from build123d import *

# Parameters (mm, degrees)
CROQUIS2_R                                           = 170
CROQUIS2_R_2                                         = 150
CROQUIS2_R_3                                         = 67.5
CROQUIS2_R_4                                         = 25
SALIENTE_EXTRUIR1_DEPTH                              = 100
CROQUIS3_R                                           = 150
CORTAR_EXTRUIR1_DEPTH                                = 50
CROQUIS4_R                                           = 67.5
CORTAR_EXTRUIR3_DEPTH                                = 80
CROQUIS5_W                                           = 15
CROQUIS5_H                                           = 35
CORTAR_EXTRUIR4_DEPTH                                = 261.384331326
AVELLANADO_PARA_TORNILLO_CON_CABEZA_AVEL_D           = 10
AVELLANADO_PARA_TORNILLO_CON_CABEZA_AVEL_CSINK_D     = 17.3
AVELLANADO_PARA_TORNILLO_CON_CABEZA_AVEL_CSINK_ANGLE = 90


with BuildPart() as part:
    # Croquis2 → Saliente-Extruir1 (new body)
    # profile 1 of 3: a face of its own
    with BuildSketch(Plane.XY):
        Circle(CROQUIS2_R)
        Circle(CROQUIS2_R_2, mode=Mode.SUBTRACT)
    # profile 2 of 3: a face of its own
    with BuildSketch(Plane.XY):
        Circle(CROQUIS2_R_2)
        Circle(CROQUIS2_R_3, mode=Mode.SUBTRACT)
    # profile 3 of 3: a face of its own
    with BuildSketch(Plane.XY):
        Circle(CROQUIS2_R_3)
        Circle(CROQUIS2_R_4, mode=Mode.SUBTRACT)
    extrude(amount=SALIENTE_EXTRUIR1_DEPTH)

    # Croquis3 → Cortar-Extruir1 (cut)
    with BuildSketch(Plane.XY):
        Circle(CROQUIS3_R)
    extrude(amount=CORTAR_EXTRUIR1_DEPTH, mode=Mode.SUBTRACT)

    # Croquis4 → Cortar-Extruir3 (cut)
    with BuildSketch(Plane.XY):
        Circle(CROQUIS4_R)
    extrude(amount=CORTAR_EXTRUIR3_DEPTH, mode=Mode.SUBTRACT)

    # Croquis5 → Cortar-Extruir4 (cut, through all)
    with BuildSketch(Plane.XY):
        with Locations((0, 17.5)):
            Rectangle(CROQUIS5_W, CROQUIS5_H)
    extrude(amount=CORTAR_EXTRUIR4_DEPTH, mode=Mode.SUBTRACT)

    # Avellanado para tornillo con cabeza avellanada de M81 (through all)
    with Locations(Plane(origin=(0, 0, 50), x_dir=(-1, 0, 0), z_dir=(0, 0, -1))):
        with Locations((0, 106.839777093)):
            CounterSinkHole(AVELLANADO_PARA_TORNILLO_CON_CABEZA_AVEL_D / 2, AVELLANADO_PARA_TORNILLO_CON_CABEZA_AVEL_CSINK_D / 2, counter_sink_angle=AVELLANADO_PARA_TORNILLO_CON_CABEZA_AVEL_CSINK_ANGLE)


solid = part.part
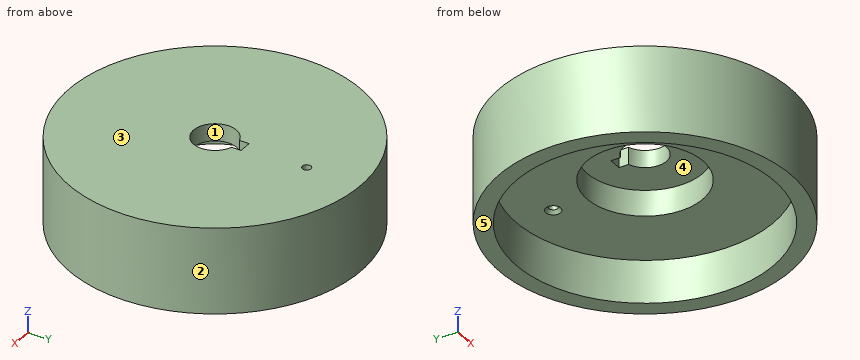
The model under review builds one solid part; all positions refer to its coordinate system, in mm. Face numbers are marked on the shaded views. A direction names the side the tool comes from. Give positions to 0.01 mm unless a question says otherwise; leave off trailing zeros. Order: outer loops, then holes, each group sorted by start corner. A loop starts at its lowest first (then second) coordinate and runs counter-clockwise, first axis right, second up. Notation, with made-up numbers: (-3.75, 1) -> (1.25, 1) arc R16 ccw to (1.25, 23) -> close; hole circle Ø11 at (6, -28). An arc over 180 degrees is marked (long way). Write item = value, one per line. Start each with the question number.
(1) For pin 1 Ø1 at (y, z) = (16.5, 78) entering from -X; pin 2 Ø1 at (x, z) = (132.5, 68.5) entering from +Y; pin 3 Ø10 at (y, z) = (-50, 23) entering from -X; pin 4 Ø6 at (x, y) = (0, 106.84) entering from +Z, all flat-tipped, find the tip position at first contact; note any pin that passes through.
(2) Draft analysis for pull direction Y (two halves, no side actions). For the marked faces 1, 2 and 3, state which applies: +Y half, -Y half, draft (parallel to the pull), parting line (faces both ways), or undercut.
(3) Take a section at D-D (x = -99). Write out the cut boundary in (y, z).
(4) Tool access review of the marked faces 4 and 5: name each direction out of +Z, -Z, +X, -X, +Y, -Y from which nothing blocks a thin tool from reaching the whole face with its end or side.
(5) Take a section at A-A (y = 0). Write out the cut boundary in (x, z), plus the area to 4 significant figures.
(6) For L1, parallel to Y at x = 0, z = 65; L2, parallel to Y at x = 0, z = 94; L3, parallel to Z at x = -98.5, y = 84.5, list the stretches that pass through material, from the lowest coordinate up. Write a range as from..to.
(7) Take a section at B-B (x = 0). Write out the cut boundary in (y, z).
(8) Take a section at C-C (z = 15). Write out the cut boundary in (x, y), plus the area to 3 significant figures.
Returned:
q1.pin_1 = -169.25
q1.pin_2 = 107.13
q1.pin_3 = -163.94
q1.pin_4 = through
q2.face_1 = undercut
q2.face_2 = parting line
q2.face_3 = draft
q3.outline = (-138.2, 0) -> (-112.69, 0) -> (-112.69, 50) -> (112.69, 50) -> (112.69, 0) -> (138.2, 0) -> (138.2, 100) -> (-138.2, 100) -> close
q4.face_4 = -Z
q4.face_5 = -Z, +X, -X, +Y, -Y
q5.outline = (-170, 0) -> (-150, 0) -> (-150, 50) -> (-67.5, 50) -> (-67.5, 80) -> (-25, 80) -> (-25, 100) -> (-170, 100) -> close; (25, 80) -> (67.5, 80) -> (67.5, 50) -> (150, 50) -> (150, 0) -> (170, 0) -> (170, 100) -> (25, 100) -> close
q5.area = 13,950 mm²
q6.L1 = -170..-67.5, 67.5..101.84, 111.84..170
q6.L2 = -170..-25, 35..101.84, 111.84..170
q6.L3 = 50..100
q7.outline = (-170, 0) -> (-150, 0) -> (-150, 50) -> (-67.5, 50) -> (-67.5, 80) -> (-25, 80) -> (-25, 100) -> (-170, 100) -> close; (35, 80) -> (67.5, 80) -> (67.5, 50) -> (98.19, 50) -> (101.84, 53.65) -> (101.84, 100) -> (35, 100) -> close; (111.84, 53.65) -> (115.49, 50) -> (150, 50) -> (150, 0) -> (170, 0) -> (170, 100) -> (111.84, 100) -> close
q8.outline = circle Ø340 at (0, 0); hole circle Ø300 at (0, 0)
q8.area = 20,100 mm²
